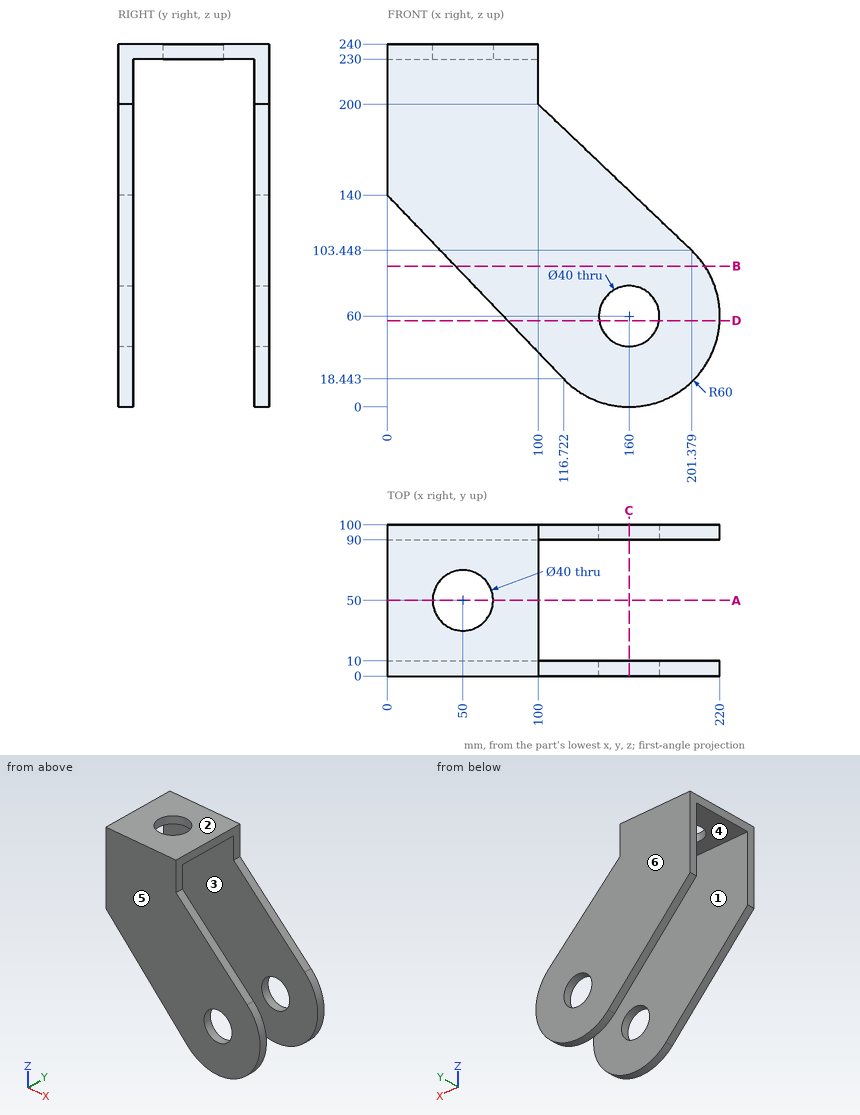
The figure shows three views and two pictorial views of one solid part (mm, origin at its lowest corner). Answer the questions. A direction names the side the tool comes from. Round coordinates to 2 decimals unless told otherwise and drop trailing zeros. Write each loop counter-clockwise with the first axis right and the second up, starting at its lowest first coordinate (ties: lowest second). Pieces come first, ordered by that corner, then holes. Notation, with made-up numbers: (64.25, 34.5) -> (108.25, 34.5) arc R15 ccw to (108.25, 61.5) -> close; hole circle Ø8 at (57.25, -11.75). An arc over 180 degrees is marked (long way). Answer as a JSON object with one key per item and string values. Group by question number.
Q1. Section C-C (x = 160) is taken. Write down the section's boundary in (y, z), plus the area to 3 significant figures.
Q2. Section D-D (z = 57) is taken. Write down the section's boundary in (x, y) (1 decimal), plus the area to 3 significant figures.
Q3. Which of the six approach directions +Z, -Z, +X, -X, +Y, -Y give full straight-line access (tool end or side, diameter ignored) to the marked faces 1 and 2?
Q4. Determine the mould class of the marked faces 3, 4, 5 and 6 for opening direction Y: pulls with the +Y half, pulls with the -Y half, needs draft (parallel to the pull), parting line crosses it, or undercut.
Q5. This flat-tipped pin is pushed along its axis until it touches: pin 1 Ø8 at (x, y) = (87, 47) entering from -Z. Where does it stop, or does it pass through?
Q6. Section B-B (z = 93) is taken. Write down the section's boundary in (x, y).
Q7. Straight lines are drawn through the part: line 1 along Y through (x, z) = (188, 71.5); line 2 along Y through (x, z) = (50, 233); line 3 along Z through (x, y) = (160, 95) (1 decimal). For each, find the intervals that lie inside material, in ascending order.
Q8. Section A-A (y = 50) is taken. Write down the section's boundary in (x, z), plus the area to 3 significant figures.
Check values:
{
 "1": {"outline": "(0, 0) -> (10, 0) -> (10, 40) -> (0, 40) -> close; (0, 80) -> (10, 80) -> (10, 142.86) -> (0, 142.86) -> close; (90, 0) -> (100, 0) -> (100, 40) -> (90, 40) -> close; (90, 80) -> (100, 80) -> (100, 142.86) -> (90, 142.86) -> close", "area": "2,060 mm^2"},
 "2": {"outline": "(79.7, 0) -> (140.2, 0) -> (140.2, 10) -> (79.7, 10) -> close; (79.7, 90) -> (140.2, 90) -> (140.2, 100) -> (79.7, 100) -> close; (179.8, 0) -> (219.9, 0) -> (219.9, 10) -> (179.8, 10) -> close; (179.8, 90) -> (219.9, 90) -> (219.9, 100) -> (179.8, 100) -> close", "area": "2,010 mm^2"},
 "3": {"face 1": "-Z, +X, -X", "face 2": "+Z, +X, -X, +Y, -Y"},
 "4": {"face 3": "undercut", "face 4": "undercut", "face 5": "pulls with the -Y half", "face 6": "pulls with the +Y half"},
 "5": {"pin 1": "z = 230"},
 "6": {"outline": "(45.13, 0) -> (210.11, 0) -> (210.11, 10) -> (45.13, 10) -> close; (45.13, 90) -> (210.11, 90) -> (210.11, 100) -> (45.13, 100) -> close"},
 "7": {"line 1": "0 to 10, 90 to 100", "line 2": "0 to 30, 70 to 100", "line 3": "0 to 40, 80 to 142.9"},
 "8": {"outline": "(0, 230) -> (30, 230) -> (30, 240) -> (0, 240) -> close; (70, 230) -> (100, 230) -> (100, 240) -> (70, 240) -> close", "area": "600 mm^2"}
}
